CAD build for the part. Positions are in the model's coordinates, mm. Give positions to 0.01 mm unless a question says otherwise; leave off trailing zeros. Loops run counter-clockwise (first coordinate to the right, second up) from the corner with the lowest first, then second, coordinate; pieces in that order, holes last.
Item 1: Saw through at A-A on x = -571.5. Give the cut face in (y, z) (3 decimals).
Item 2: Drop flat-ended pins along their axis: P1, Ø12.5, axis at x = -139.7, z = 0, coming from the +Y side; P2, Ø12.5, axis at x = -190.5, y = 0, coming from the +Z side. Give the stop position or say it passes through.
Item 3: Probe probe 1 along Z at (x, y) = (-72, -12); probe 2 along Y at (x, z) = (-204.5, 10.5) (3 decimals); probe 3 along Z at (x, y) = (-165.1, -14.9) (3 decimals). List the from-to ranges inside material, lowest first.
Item 4: Saw through at B-B on x = -433.5. Give the cut face in (y, z) (3 decimals), plus the area to 3 significant figures.
Item 5: Saw through at C-C on x = -190. Give the cut face in (y, z) (3 decimals), plus the area to 3 significant figures.
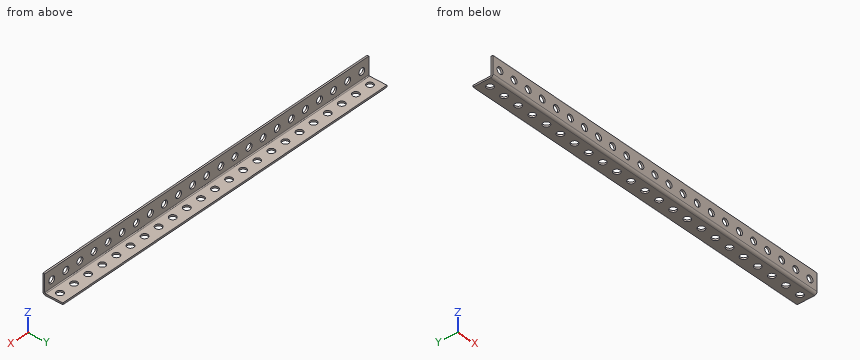
from build123d import *

# Parameters (mm, degrees)
BOSS_EXTRUDE1_DEPTH      = 609.6
BOSS_EXTRUDE1_DEPTH_BACK = 609.6
SKETCH5_R                = 5.334
CUT_EXTRUDE1_DEPTH       = 16.875
SKETCH6_R                = 5.334
CUT_EXTRUDE2_DEPTH       = 16.875
LPATTERN1_COUNT          = 48
LPATTERN1_PITCH          = 25.4
SKETCH7_W                = 635
SKETCH7_H                = 31.75
CUT_EXTRUDE3_DEPTH       = 70


with BuildPart() as part:
    # Sketch4 → Boss-Extrude1 (new body, two sides)
    with BuildSketch(Plane(origin=(0, 0, 0), x_dir=(0, 0, -1), z_dir=(1, 0, 0))) as boss_extrude1_sk:
        with BuildLine():
            Line((-15.875, -13.1318), (11.7602, -13.1318))
            ThreePointArc((11.7602, -13.1318), (12.730067661, -12.730067661), (13.1318, -11.7602))
            Line((13.1318, -11.7602), (13.1318, 15.875))
            Line((13.1318, 15.875), (15.875, 15.875))
            Line((15.875, 15.875), (15.875, -11.7602))
            ThreePointArc((15.875, -11.7602), (14.669802983, -14.669802983), (11.7602, -15.875))
            Line((11.7602, -15.875), (-15.875, -15.875))
            Line((-15.875, -15.875), (-15.875, -13.1318))
        make_face()
    extrude(amount=BOSS_EXTRUDE1_DEPTH)
    extrude(boss_extrude1_sk.sketch, amount=-BOSS_EXTRUDE1_DEPTH_BACK)

    # Sketch5 → Cut-Extrude1 (cut, through all)
    with BuildSketch(Plane.XY):
        with Locations((596.9, 0)):
            Circle(SKETCH5_R)
    cut_extrude1 = extrude(amount=-CUT_EXTRUDE1_DEPTH, mode=Mode.SUBTRACT)

    # Sketch6 → Cut-Extrude2 (cut, through all)
    with BuildSketch(Plane(origin=(0, 0, 0), x_dir=(1, 0, 0), z_dir=(0, 1, 0))):
        with Locations((596.9, 0)):
            Circle(SKETCH6_R)
    cut_extrude2 = extrude(amount=-CUT_EXTRUDE2_DEPTH, mode=Mode.SUBTRACT)

    # LPattern1: Cut-Extrude1, Cut-Extrude2 ×48
    with Locations(*[(-i * LPATTERN1_PITCH, 0, 0) for i in range(1, LPATTERN1_COUNT)]):
        add(cut_extrude1, mode=Mode.SUBTRACT)
        add(cut_extrude2, mode=Mode.SUBTRACT)

    # Sketch7 → Cut-Extrude3 (cut)
    with BuildSketch(Plane(origin=(0, 0, -15.875), x_dir=(-1, 0, 0), z_dir=(0, 0, -1))):
        with Locations((-292.1, 0)):
            Rectangle(SKETCH7_W, SKETCH7_H)
    extrude(amount=-CUT_EXTRUDE3_DEPTH, mode=Mode.SUBTRACT)


solid = part.part
Results below:
1. outline: (-15.875, -11.76) arc R4.115 ccw to (-11.76, -15.875) - (-5.334, -15.875) - (-5.334, -13.132) - (-11.76, -13.132) arc R1.372 cw to (-13.132, -11.76) - (-13.132, -5.334) - (-15.875, -5.334) - close; (-15.875, 5.334) - (-13.132, 5.334) - (-13.132, 15.875) - (-15.875, 15.875) - close; (5.334, -15.875) - (15.875, -15.875) - (15.875, -13.132) - (5.334, -13.132) - close
2. P1: stops at y = -13.13
2. P2: stops at z = -13.13
3. probe 1: z = -15.87 to -13.11
3. probe 2: y = -15.875 to -13.132
3. probe 3: z = -14.42 to -5.334, 5.334 to 15.875
4. outline: (-15.875, -11.76) arc R4.115 ccw to (-11.76, -15.875) - (15.875, -15.875) - (15.875, -13.132) - (-11.76, -13.132) arc R1.372 cw to (-13.132, -11.76) - (-13.132, 15.875) - (-15.875, 15.875) - close
4. area: 163 mm2
5. outline: (-15.875, -11.76) arc R4.115 ccw to (-11.76, -15.875) - (-5.311, -15.875) - (-5.311, -13.132) - (-11.76, -13.132) arc R1.372 cw to (-13.132, -11.76) - (-13.132, -5.311) - (-15.875, -5.311) - close; (-15.875, 5.311) - (-13.132, 5.311) - (-13.132, 15.875) - (-15.875, 15.875) - close; (5.311, -15.875) - (15.875, -15.875) - (15.875, -13.132) - (5.311, -13.132) - close
5. area: 105 mm2
